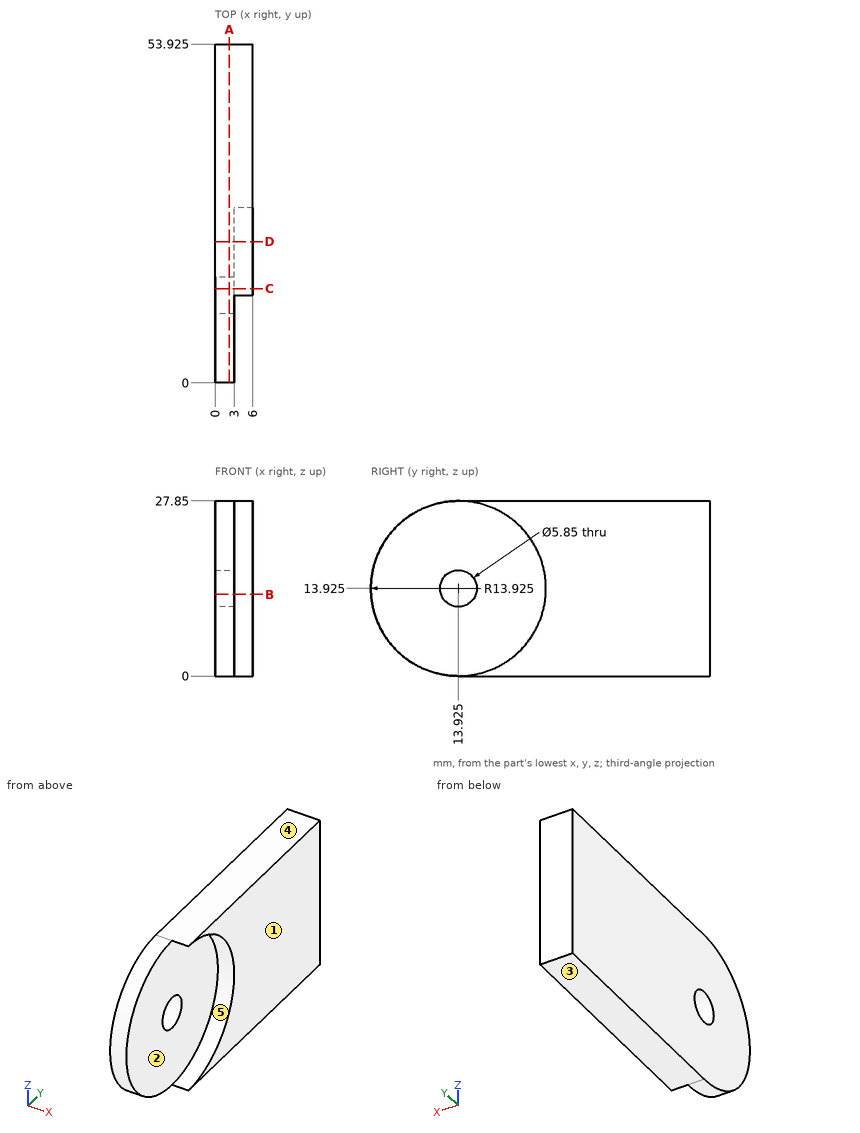
Drawing for the job (mm, zero at the part's lowest x, y, z). A direction names the side the tool comes from. Give positions to 0.01 mm unless a question says otherwise; leave off trailing zeros. Write each loop counter-clockwise with the first axis right and the second up, starting at its lowest first coordinate (ties: lowest second). Pieces come first, ordered by that corner, then holes. Notation, with made-up numbers: M -3,26 L 11,26 A15 ccw 11,31 Z; hole C 6.25,56.25 d6. An arc over 180 degrees is marked long. Use CSV: the item, a comma, the result in double quotes.
Item 1: Slice it at B-B on z = 13. Write the cut outline in (x, y) (3 decimals), plus the area to 3 significant figures.
Taken from the geometry:
outline,"M 0,0.031 L 3,0.031 L 3,11.15 L 0,11.15 Z; M 0,16.7 L 3,16.7 L 3,27.819 L 6,27.819 L 6,53.925 L 0,53.925 Z"
area,"223 mm²"
Item 2: Pin check, flat tips, straight feed: P1, Ø8.5, axis at y = 20.5, z = 16, coming from the +X side; P2, Ø3, axis at x = 3, z = 21, coming from the -Y side; P3, Ø3.5, axis at y = 13.925, z = 13.925, coming from the +X side. Stop position of each tip, or through.
Taken from the geometry:
P1,"stops at x = 3"
P2,"stops at y = 1.16"
P3,"passes through"
Item 3: Slice it at A-A on x = 2.25. Write the cut outline in (y, z) (3 decimals).
Taken from the geometry:
outline,"M 13.925,0 L 53.925,0 L 53.925,27.85 L 13.925,27.85 A13.925 ccw Z; hole C 13.925,13.925 d5.85"
Item 4: Pull direction Z, two halves, no side cores. Call the marked faces 1, 2 and 3: +Z half, -Z half, draft (parallel to the pull), parting line (faces both ways), or undercut.
Taken from the geometry:
face 1,"draft"
face 2,"undercut"
face 3,"-Z half"
Item 5: Slice it at D-D on y = 22.5. Write the cut outline in (x, z).
Taken from the geometry:
outline,"M 0,0 L 6,0 L 6,2.95 L 3,2.95 L 3,24.9 L 6,24.9 L 6,27.85 L 0,27.85 Z"
Item 6: Slice it at C-C on y = 15. Write the cut outline in (x, z), plus the area to 3 significant figures.
Taken from the geometry:
outline,"M 0,0 L 6,0 L 6,0.04 L 3,0.04 L 3,11.2 L 0,11.2 Z; M 0,16.65 L 3,16.65 L 3,27.81 L 6,27.81 L 6,27.85 L 0,27.85 Z"
area,"67.5 mm²"
Item 7: Which spindle directions (+Z, -Z, +X, -X, +Y, -Y) get a long thin tool onto all of the face, cutting with end or side? Do the marked faces 4 and 5. Say none if no direction does.
Taken from the geometry:
face 4,"+Z, +X, -X, +Y, -Y"
face 5,"+X, -Y"
Item 8: Drill centre lines: probe 1 along X at (y, z) = (2, 18.25); probe 2 along Z at (x, y) = (3.3, 21); probe 3 along Z at (x, y) = (0.6, 13.5). Where is each one in solid material? Low to high.
Taken from the geometry:
probe 1,"x = 0 to 3"
probe 2,"z = 0 to 1.93, 25.92 to 27.85"
probe 3,"z = 0.01 to 11.03, 16.82 to 27.84"
